from build123d import *

# Parameters (mm, degrees)
BOSS_EXTRUDE1_DEPTH = 2.95


with BuildPart() as part:
    # Sketch1 → Boss-Extrude1 (new body)
    with BuildSketch(Plane(origin=(0, 0, 0), x_dir=(1, 0, 0), z_dir=(0, 1, 0))):
        with BuildLine():
            Line((5, -75), (5, -69.409830056))
            ThreePointArc((5, -69.409830056), (0, -67.5), (-5, -69.409830056))
            Line((-5, -69.409830056), (-5, -75))
            Line((-5, -75), (-2.65, -75))
            Line((-2.65, -75), (-2.65, -73.470021787))
            Line((-2.65, -73.470021787), (0, -71.940043573))
            Line((0, -71.940043573), (2.65, -73.470021787))
            Line((2.65, -73.470021787), (2.65, -75))
            Line((2.65, -75), (5, -75))
        make_face()
        with BuildLine():
            Line((-5, -75), (-5, -69.409830056))
            ThreePointArc((-5, -69.409830056), (-7.372988698, -76.374422666), (-2.65, -82.016231182))
            Line((-2.65, -82.016231182), (-2.65, -76.529978213))
            Line((-2.65, -76.529978213), (-2.65, -75))
            Line((-2.65, -75), (-5, -75))
        make_face()
        with BuildLine():
            ThreePointArc((7.5, -75), (6.846531969, -71.938137822), (5, -69.409830056))
            Line((5, -69.409830056), (5, -75))
            Line((5, -75), (2.65, -75))
            Line((2.65, -75), (2.65, -76.529978213))
            Line((2.65, -76.529978213), (2.65, -82.016231182))
            ThreePointArc((2.65, -82.016231182), (6.16948134, -79.264680527), (7.5, -75))
        make_face()
        with BuildLine():
            Line((5, -69.409830056), (5, -5.590169944))
            ThreePointArc((5, -5.590169944), (0, -7.5), (-5, -5.590169944))
            Line((-5, -5.590169944), (-5, -69.409830056))
            ThreePointArc((-5, -69.409830056), (0, -67.5), (5, -69.409830056))
        make_face()
        with BuildLine():
            Line((2.65, 1.529978213), (2.65, 0))
            Line((2.65, 0), (5, 0))
            Line((5, 0), (5, -5.590169944))
            ThreePointArc((5, -5.590169944), (6.846531969, -3.061862178), (7.5, 0))
            ThreePointArc((7.5, 0), (-3.061862178, 6.846531969), (-5, -5.590169944))
            Line((-5, -5.590169944), (-5, 0))
            Line((-5, 0), (-2.65, 0))
            Line((-2.65, 0), (-2.65, 1.529978213))
            Line((-2.65, 1.529978213), (0, 3.059956427))
            Line((0, 3.059956427), (2.65, 1.529978213))
        make_face()
        with BuildLine():
            Line((2.65, -1.529978213), (0, -3.059956427))
            Line((0, -3.059956427), (-2.65, -1.529978213))
            Line((-2.65, -1.529978213), (-2.65, 0))
            Line((-2.65, 0), (-5, 0))
            Line((-5, 0), (-5, -5.590169944))
            ThreePointArc((-5, -5.590169944), (0, -7.5), (5, -5.590169944))
            Line((5, -5.590169944), (5, 0))
            Line((5, 0), (2.65, 0))
            Line((2.65, 0), (2.65, -1.529978213))
        make_face()
    extrude(amount=BOSS_EXTRUDE1_DEPTH)


solid = part.part
Could you check a few things on this model? Use its own coordinates, in mm. A direction names the side the tool comes from. Give positions to 0.01 mm unless a question says otherwise; leave off trailing zeros. Order: outer loops, then holes, each group sorted by start corner. A loop starts at its lowest first (then second) coordinate and runs counter-clockwise, first axis right, second up.
1. Suppose I cut it at B-B (x = 1.5). List the corners of the cut face in (y, z) for me.
2. Will these pins go through, and if not, where does the flat tip stop? P1, Ø1.5, axis at x = -1.5, y = 2, coming from the +Z side; P2, Ø1, axis at y = 0.5, z = 49, coming from the +X side; P3, Ø2, axis at x = -5, z = 38, coming from the -Y side; P4, Ø1.5, axis at y = 1.5, z = 24, coming from the -X side.
3. Suppose I cut it at A-A (y = 2.1). List the corners of the cut face in (x, z) for me, plus the area to 3 significant figures.
4. Suppose I cut it at C-C (z = 54). List the corners of the cut face in (x, y) for me.
5. I need wall thicknesses on L1, parallel to Z at x = 6, y = 2.35; L2, parallel to X at y = 0.6, z = 9; L3, parallel to Z at x = 0.75, y = 0.5. Which ranges of each line are inside material? Lowest first, please.
6. For faces 5 (the flat face through (0, 0, 37)), 6 (the flat face through (-5, 1, 37)), 7 (the flat face through (-1.344, 1.454, 72.716)), 8 (the flat face through (-1.306, 1.454, 2.306)), which set-ups out of +Z, -Z, +X, -X, +Y, -Y let a thin tool reach every point of the face, with its end or its side?
7. We'd pull the mould along X, two halves only. Please class faces 1 (the flat face through (5, 1, 38)), 2 (the cylindrical face through (-7.39, 1.45, 76.27)), 3 (the flat face through (2.65, 1, 78)), 4 (the flat face through (0, 2.95, 37)): pulls with the +X half, pulls with the -X half, needs draft (parallel to the pull), parting line crosses it, or undercut.
Solved:
1. outline: (0, -7.35) - (2.95, -7.35) - (2.95, -2.19) - (0, -2.19) - close; (0, 2.19) - (2.95, 2.19) - (2.95, 72.81) - (0, 72.81) - close
2. P1: stops at z = 73.24
2. P2: stops at x = 5
2. P3: stops at y = 0
2. P4: stops at x = -5
3. outline: (-5, 5.59) arc R7.5 ccw (long way) to (5, 5.59) - (5, 69.41) arc R7.5 ccw to (2.65, 82.02) - (2.65, 73.47) - (0, 71.94) - (-2.65, 73.47) - (-2.65, 82.02) arc R7.5 ccw to (-5, 69.41) - close; hole (-2.65, -1.53) - (0, -3.06) - (2.65, -1.53) - (2.65, 1.53) - (0, 3.06) - (-2.65, 1.53) - close
3. area: 890 mm2
4. outline: (-5, 0) - (5, 0) - (5, 2.95) - (-5, 2.95) - close
5. L1: z = -4.5 to 4.5, 70.5 to 79.5
5. L2: x = -5 to 5
5. L3: z = -7.46 to -2.63, 2.63 to 72.37
6. face 5: +Z, -Z, +X, -X, -Y
6. face 6: -X, +Y, -Y
6. face 7: +Z, +Y, -Y
6. face 8: +Y, -Y
7. face 1: pulls with the +X half
7. face 2: pulls with the -X half
7. face 3: undercut
7. face 4: needs draft
